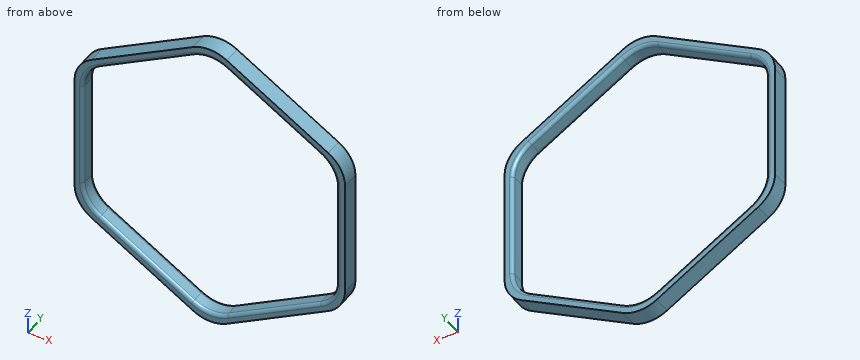
```python
from build123d import *

# Parameters (mm, degrees)
ESTRUSIONE_SOTTILE1_DEPTH = 5
RACCORDO1_R               = 10
RACCORDO2_R               = 1


with BuildPart() as part:
    # Schizzo2 → Estrusione-Sottile1 (new body)
    with BuildSketch(Plane(origin=(0, 0, 0), x_dir=(1, 0, 0), z_dir=(0, 1, 0))):
        Polygon((40, 23.094010768), (0, 46.188021535), (-40, 23.094010768), (-40, -23.094010768), (0, -46.188021535), (40, -23.094010768), align=None)
        Polygon((37.5, 21.650635095), (0, 43.301270189), (-37.5, 21.650635095), (-37.5, -21.650635095), (0, -43.301270189), (37.5, -21.650635095), align=None, mode=Mode.SUBTRACT)
    extrude(amount=ESTRUSIONE_SOTTILE1_DEPTH)

    # Raccordo1
    raccordo1_edges = [part.edges().sort_by_distance(p)[0] for p in [
        (37.5, 2.5, 21.650635095),
        (37.5, 2.5, -21.650635095),
        (0, 2.5, -43.301270189),
        (-37.5, 2.5, -21.650635095),
        (-37.5, 2.5, 21.650635095),
        (0, 2.5, 43.301270189),
        (40, 2.5, 23.094010768),
        (0, 2.5, 46.188021535),
        (-40, 2.5, 23.094010768),
        (-40, 2.5, -23.094010768),
        (0, 2.5, -46.188021535),
        (40, 2.5, -23.094010768),
    ]]
    fillet(raccordo1_edges, radius=RACCORDO1_R)

    # Raccordo2
    raccordo2_edges = [part.edges().sort_by_distance(p)[0] for p in [
        (37.5, 0, 0),
        (18.75, 0, -32.475952642),
        (-18.75, 0, -32.475952642),
        (-37.5, 0, 0),
        (-18.75, 0, 32.475952642),
        (18.75, 0, 32.475952642),
        (18.75, 5, -32.475952642),
        (37.5, 5, 0),
        (18.75, 5, 32.475952642),
        (-18.75, 5, 32.475952642),
        (-37.5, 5, 0),
        (-18.75, 5, -32.475952642),
        (36.160254038, 0, 20.877132403),
        (36.160254038, 5, 20.877132403),
        (0, 0, 41.754264805),
        (0, 5, 41.754264805),
        (36.160254038, 0, -20.877132403),
        (36.160254038, 5, -20.877132403),
        (0, 0, -41.754264805),
        (0, 5, -41.754264805),
        (-36.160254038, 0, -20.877132403),
        (-36.160254038, 5, -20.877132403),
        (-36.160254038, 0, 20.877132403),
        (-36.160254038, 5, 20.877132403),
    ]]
    fillet(raccordo2_edges, radius=RACCORDO2_R)


solid = part.part
```
Read the model definition and answer for the solid it produces. Units are mm, in the model's axes. Give positions to 0.01 mm unless a question says otherwise; leave off trailing zeros. Order: outer loops, then holes, each group sorted by start corner. A loop starts at its lowest first (then second) coordinate and runs counter-clockwise, first axis right, second up.
(1) Straight lines are drawn through the part: L1, parallel to X at y = 1.15, z = -8.5; L2, parallel to X at y = 3.4, z = -34; L3, parallel to Z at x = -8.5, y = 1.25. For each, find the intervals that lie inside material, in ascending order.
(2) Find section A-A (y = 3.05). Give the vertices of the cut face in (x, z), plus the area to 3 significant figures.
(3) Given pin 1 (2 mm diameter, centred on y = 3.5, z = -20, fed in from +X); pin 2 (10 mm diameter, centred on x = -30.5, z = -12.5, fed in from +Y), each flat-ended and moving along its own axis, determine where each tip first touches the part or whether it passes through.
(4) Find section B-B (z = -7). Give the vertices of the cut face in (x, y), plus the area to 3 significant figures.
Result sheet:
1. L1: x = -40 to -37.5, 37.5 to 40
1. L2: x = -21.11 to -16.11, 16.11 to 21.11
1. L3: z = -41.28 to -38.39, 38.39 to 41.28
2. outline: (-40, -17.32) arc R10 ccw to (-35, -25.98) - (-5, -43.3) arc R10 ccw to (5, -43.3) - (35, -25.98) arc R10 ccw to (40, -17.32) - (40, 17.32) arc R10 ccw to (35, 25.98) - (5, 43.3) arc R10 ccw to (-5, 43.3) - (-35, 25.98) arc R10 ccw to (-40, 17.32) - close; hole (-37.5, -15.88) arc R10 ccw to (-32.5, -24.54) - (-5, -40.41) arc R10 ccw to (5, -40.41) - (32.5, -24.54) arc R10 ccw to (37.5, -15.88) - (37.5, 15.88) arc R10 ccw to (32.5, 24.54) - (5, 40.41) arc R10 ccw to (-5, 40.41) - (-32.5, 24.54) arc R10 ccw to (-37.5, 15.88) - close
2. area: 671 mm2
3. pin 1: stops at x = 39.86
3. pin 2: passes through
4. outline: (-40, 0) - (-38.5, 0) arc R1 ccw to (-37.5, 1) - (-37.5, 4) arc R1 ccw to (-38.5, 5) - (-40, 5) - close; (37.5, 1) arc R1 ccw to (38.5, 0) - (40, 0) - (40, 5) - (38.5, 5) arc R1 ccw to (37.5, 4) - close
4. area: 24.1 mm2
